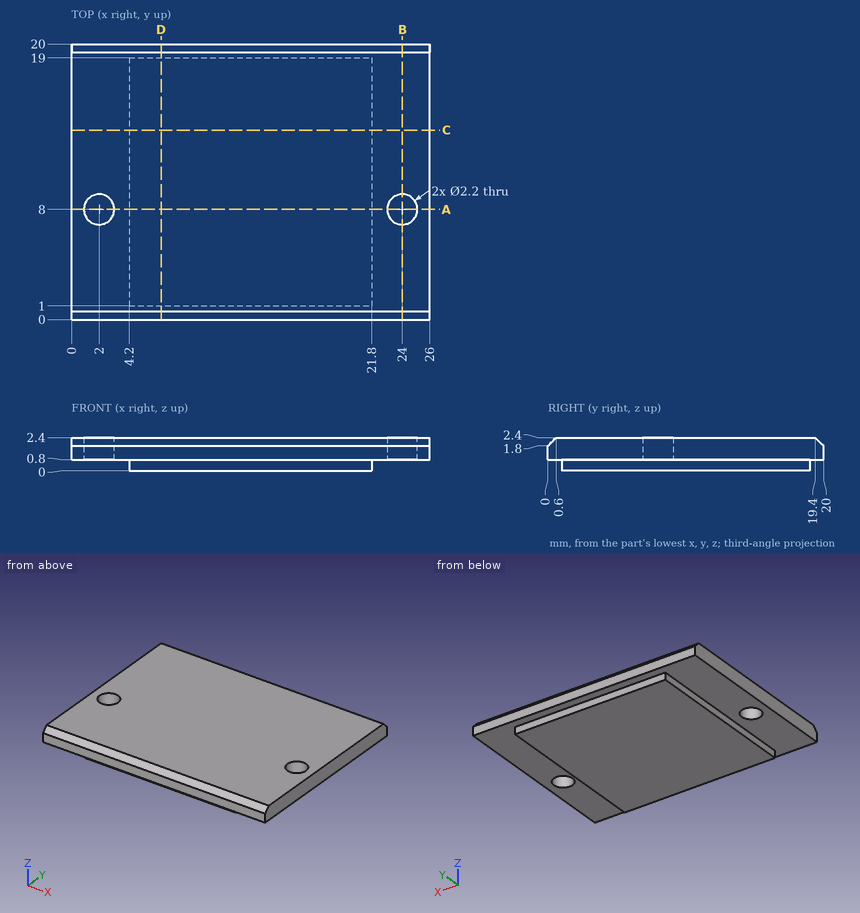
Input: dimensioned drawing with shaded views. Units: mm. Origin: part minimum x, y, z. Coordinates: 2 decimals unless noted, no trailing zeros. Loops run counter-clockwise (first coordinate to the right, second up) from the corner with the lowest first, then second, coordinate; pieces in that order, holes last. Notation, with made-up numbers: (-23.75, -14.5) - (33.25, -14.5) arc R16 ccw to (33.25, 8.5) - close; hole circle Ø7 at (14.5, -2). An arc over 180 degrees is marked (long way). One line per question, with ' | ' between items. Start each with the question number.
(1) Cut plane D-D on x = 6.5. Output: boundary loops of the cut face in (y, z), and give its area (3 significant figures).
(2) Cut plane A-A on y = 8. Output: boundary loops of the cut face in (x, z), and give its area (3 significant figures).
(3) Cut plane B-B on x = 24. Output: boundary loops of the cut face in (y, z), and give its area (3 significant figures).
(4) Cut plane C-C on y = 13.75. Output: boundary loops of the cut face in (x, z).
(5) Ray query, L1, parallel to Y at x = 24, z = 1.7; L2, parallel to Z at x = 3.5, y = 10; L3, parallel to Y at x = 24, z = 2. Return the intervals inside material, ascending. Write a range as from..to.
(6) First-contact query: pin 1 (1.3 mm diameter, centred on x = 24, y = 8, fed in from -Z). Flat tip, straight axial feed; report the tip coordinate or a pass-through.
Here are the results:
1) outline: (0, 0.8) - (1, 0.8) - (1, 0) - (19, 0) - (19, 0.8) - (20, 0.8) - (20, 1.8) - (19.4, 2.4) - (0.6, 2.4) - (0, 1.8) - close | area: 46.0 mm²
2) outline: (0, 0.8) - (0.9, 0.8) - (0.9, 2.4) - (0, 2.4) - close; (3.1, 0.8) - (4.2, 0.8) - (4.2, 0) - (21.8, 0) - (21.8, 0.8) - (22.9, 0.8) - (22.9, 2.4) - (3.1, 2.4) - close; (25.1, 0.8) - (26, 0.8) - (26, 2.4) - (25.1, 2.4) - close | area: 48.6 mm²
3) outline: (0, 0.8) - (6.9, 0.8) - (6.9, 2.4) - (0.6, 2.4) - (0, 1.8) - close; (9.1, 0.8) - (20, 0.8) - (20, 1.8) - (19.4, 2.4) - (9.1, 2.4) - close | area: 28.1 mm²
4) outline: (0, 0.8) - (4.2, 0.8) - (4.2, 0) - (21.8, 0) - (21.8, 0.8) - (26, 0.8) - (26, 2.4) - (0, 2.4) - close
5) L1: 0..6.9, 9.1..20 | L2: 0.8..2.4 | L3: 0.2..6.9, 9.1..19.8
6) pin 1: through
